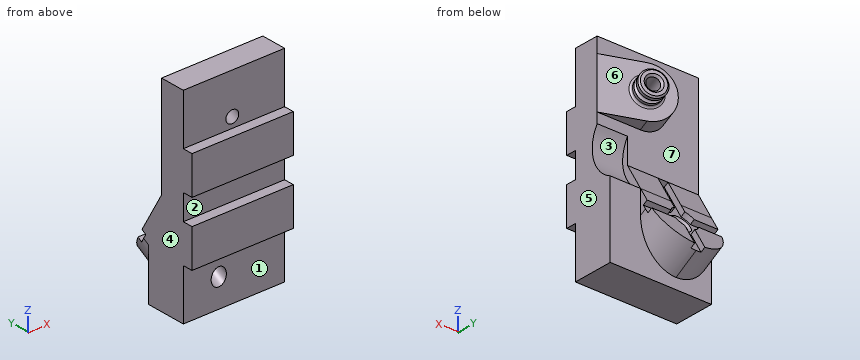
```python
from build123d import *

# Parameters (mm, degrees)
BOSS_EXTRUDE1_DEPTH     = 100
CUT_EXTRUDE1_DEPTH      = 30
BOSS_EXTRUDE2_START     = -15
BOSS_EXTRUDE2_DEPTH     = 50
CUT_EXTRUDE2_REACH      = 226.87
SKETCH5_R               = 12.5
BOSS_EXTRUDE4_DEPTH     = 15
SKETCH7_R               = 6
CUT_EXTRUDE4_DEPTH      = 228.547988513
FILLET1_R               = 2
CHAMFER1_SIZE           = 2
CHAMFER2_SIZE           = 1.5
BOSS_EXTRUDE5_DEPTH     = 70
CUT_EXTRUDE5_REACH      = 232.227
CUT_EXTRUDE6_DEPTH      = 5
CUT_EXTRUDE7_DEPTH      = 230.919504684
CUT_EXTRUDE7_DEPTH_BACK = 230.919504684
SKETCH17_R              = 7.5
CHAMFER3_SIZE           = 2


with BuildPart() as part:
    # Sketch1 → Boss-Extrude1 (new body)
    with BuildSketch(Plane(origin=(0, 0, 0), x_dir=(0, 0, -1), z_dir=(1, 0, 0))):
        Polygon((0, 0), (50, 0), (50, -10), (87.5, -10), (87.5, 0), (112.5, 0), (112.5, -10), (150, -10), (150, 0), (200, 0), (200, 40), (125.980762114, 40), (100, 25), (0, 25), align=None)
    extrude(amount=BOSS_EXTRUDE1_DEPTH)

    # Sketch2 → Cut-Extrude1 (cut)
    with BuildSketch(Plane(origin=(100, 0, 0), x_dir=(0, 0, -1), z_dir=(1, 0, 0))):
        with BuildLine():
            Line((100, 25), (75, 25))
            ThreePointArc((75, 25), (103.939266476, 20.77821286), (125.980762114, 40))
            Line((125.980762114, 40), (100, 25))
        make_face()
    extrude(amount=-CUT_EXTRUDE1_DEPTH, mode=Mode.SUBTRACT)

    # Sketch3 → Boss-Extrude2 (add)
    with BuildSketch(Plane.XY.offset(BOSS_EXTRUDE2_START)):
        Polygon((100, 25), (30.828444789, 25), (38.919979649, 47.231309316), align=None)
    extrude(amount=-BOSS_EXTRUDE2_DEPTH)

    # Cut-Extrude2: up to this plane
    cut_extrude2_end = Plane(origin=(100, 25, 0), z_dir=(0, -1, 0))
    # Sketch4 → Cut-Extrude2 (cut, up to the surface)
    with BuildSketch(Plane(origin=(19.732622965, 54.214936023, 0), x_dir=(0.9396926207859106, -0.3420201433256628, 0), z_dir=(0.34202014332566283, 0.9396926207859106, 0)), mode=Mode.PRIVATE) as cut_extrude2_sk1:
        with BuildLine():
            ThreePointArc((20.418758495, 40), (27.741088966, 57.67766953), (45.418758495, 65))
            Line((45.418758495, 65), (20.418758495, 65))
            Line((20.418758495, 65), (20.418758495, 40))
        make_face()
    cut_extrude2_tool1 = split(extrude(cut_extrude2_sk1.sketch, amount=-CUT_EXTRUDE2_REACH, mode=Mode.PRIVATE), bisect_by=cut_extrude2_end, keep=Keep.BOTH, mode=Mode.PRIVATE)
    add(cut_extrude2_tool1.solids().sort_by_distance((44.16741, 45.321401, -59.415802))[0], mode=Mode.SUBTRACT)
    # Sketch4 → Cut-Extrude2 (cut, up to the surface)
    with BuildSketch(Plane(origin=(19.732622965, 54.214936023, 0), x_dir=(0.9396926207859106, -0.3420201433256628, 0), z_dir=(0.34202014332566283, 0.9396926207859106, 0)), mode=Mode.PRIVATE) as cut_extrude2_sk2:
        with BuildLine():
            ThreePointArc((45.418758495, 15), (27.741088966, 22.32233047), (20.418758495, 40))
            Line((20.418758495, 40), (20.418758495, 15))
            Line((20.418758495, 15), (45.418758495, 15))
        make_face()
    cut_extrude2_tool2 = split(extrude(cut_extrude2_sk2.sketch, amount=-CUT_EXTRUDE2_REACH, mode=Mode.PRIVATE), bisect_by=cut_extrude2_end, keep=Keep.BOTH, mode=Mode.PRIVATE)
    add(cut_extrude2_tool2.solids().sort_by_distance((44.16741, 45.321401, -20.584198))[0], mode=Mode.SUBTRACT)

    # Sketch5 → Boss-Extrude4 (add)
    with BuildSketch(Plane(origin=(19.732622965, 54.214936023, 0), x_dir=(0.9396926207859106, -0.3420201433256628, 0), z_dir=(0.34202014332566283, 0.9396926207859106, 0))):
        with Locations(Location((45.418758495, 40, 0), (0, 0, 180))):
            Circle(SKETCH5_R)
    extrude(amount=BOSS_EXTRUDE4_DEPTH)

    # Sketch7 → Cut-Extrude4 (cut, through all)
    with BuildSketch(Plane(origin=(24.862925115, 68.310325335, 0), x_dir=(0.9396926207859105, -0.3420201433256629, 0), z_dir=(0.34202014332566294, 0.9396926207859106, 0))):
        with Locations(Location((45.418758495, 40, 0), (0, 0, 180))):
            Circle(SKETCH7_R)
    extrude(amount=-CUT_EXTRUDE4_DEPTH, mode=Mode.SUBTRACT)

    # Fillet1
    fillet1_edges = [part.edges().sort_by_distance(p)[0] for p in [
        (74.158452928, 34.405553941, -40),
    ]]
    fillet(fillet1_edges, radius=FILLET1_R)

    # Chamfer1
    chamfer1_edges = [part.edges().sort_by_distance(p)[0] for p in [
        (73.180753043, 50.724074185, -40),
    ]]
    chamfer(chamfer1_edges, length=CHAMFER1_SIZE)

    # Sketch11 → Cut-Revolve1 (revolve, cut)
    with BuildSketch(Plane(origin=(42.679672203, -15.53413029, 0), x_dir=(0.34202014332566294, 0.9396926207859105, 0), z_dir=(0.9396926207859105, -0.342020143325663, 0)), mode=Mode.PRIVATE) as cut_revolve1_sk:
        with BuildLine():
            Line((67.694329852, -27.5), (62.694329852, -27.5))
            ThreePointArc((62.694329852, -27.5), (65.194329852, -30), (67.694329852, -27.5))
        make_face()
    revolve(cut_revolve1_sk.sketch.rotate(Axis((43.396560119, -13.564496931, -40), (0.34202014332566283, 0.9396926207859105, 0)), 90), axis=Axis((43.396560119, -13.564496931, -40), (0.34202014332566283, 0.9396926207859105, 0)), mode=Mode.SUBTRACT)

    # Chamfer2
    chamfer2_edges = [part.edges().sort_by_distance(p)[0] for p in [
        (79.288755078, 48.500943253, -40),
    ]]
    chamfer(chamfer2_edges, length=CHAMFER2_SIZE)

    # Sketch13 → Boss-Extrude5 (add)
    with BuildSketch(Plane.ZY):
        Polygon((-125.980762114, 40), (-173.612159322, 67.5), (-189.489291724, 40), align=None)
    extrude(amount=-BOSS_EXTRUDE5_DEPTH)

    # Cut-Extrude5: up to this plane
    cut_extrude5_end = Plane(origin=(100, 40, -200), z_dir=(0, -1, 0))
    # Sketch14 → Cut-Extrude5 (cut, up to the surface)
    with BuildSketch(Plane(origin=(0, -24.551270189, -14.174682453), x_dir=(1, 0, 0), z_dir=(0, 0.8660254037844378, 0.5000000000000016)), mode=Mode.PRIVATE) as cut_extrude5_sk1:
        with BuildLine():
            Line((70, 184.102540378), (35, 184.102540378))
            ThreePointArc((35, 184.102540378), (59.748737342, 173.85127772), (70, 149.102540378))
            Line((70, 149.102540378), (70, 184.102540378))
        make_face()
    cut_extrude5_tool1 = split(extrude(cut_extrude5_sk1.sketch, amount=-CUT_EXTRUDE5_REACH, mode=Mode.PRIVATE), bisect_by=cut_extrude5_end, keep=Keep.BOTH, mode=Mode.PRIVATE)
    add(cut_extrude5_tool1.solids().sort_by_distance((62.182122, 63.591061, -166.841678))[0], mode=Mode.SUBTRACT)
    # Sketch14 → Cut-Extrude5 (cut, up to the surface)
    with BuildSketch(Plane(origin=(0, -24.551270189, -14.174682453), x_dir=(1, 0, 0), z_dir=(0, 0.8660254037844378, 0.5000000000000016)), mode=Mode.PRIVATE) as cut_extrude5_sk2:
        with BuildLine():
            Line((0, 184.102540378), (0, 149.102540378))
            ThreePointArc((0, 149.102540378), (10.251262658, 173.85127772), (35, 184.102540378))
            Line((35, 184.102540378), (0, 184.102540378))
        make_face()
    cut_extrude5_tool2 = split(extrude(cut_extrude5_sk2.sketch, amount=-CUT_EXTRUDE5_REACH, mode=Mode.PRIVATE), bisect_by=cut_extrude5_end, keep=Keep.BOTH, mode=Mode.PRIVATE)
    add(cut_extrude5_tool2.solids().sort_by_distance((7.817878, 63.591061, -166.841678))[0], mode=Mode.SUBTRACT)

    # Sketch15 → Cut-Extrude6 (cut)
    with BuildSketch(Plane(origin=(0, -24.551270189, -14.174682453), x_dir=(1, 0, 0), z_dir=(0, 0.8660254037844378, 0.5000000000000016))):
        with BuildLine():
            ThreePointArc((40, 183.74355653), (35, 184.102540378), (30, 183.74355653))
            Line((30, 183.74355653), (30, 160.558979616))
            ThreePointArc((30, 160.558979616), (26.161165235, 157.941375143), (23.543560763, 154.102540378))
            Line((23.543560763, 154.102540378), (0.358983849, 154.102540378))
            ThreePointArc((0.358983849, 154.102540378), (0.08986132, 151.608975566), (0, 149.102540378))
            Line((0, 149.102540378), (0, 144.102540378))
            Line((0, 144.102540378), (23.543560763, 144.102540378))
            ThreePointArc((23.543560763, 144.102540378), (26.161165235, 140.263705614), (30, 137.646101141))
            Line((30, 137.646101141), (30, 99.102540378))
            Line((30, 99.102540378), (40, 99.102540378))
            Line((40, 99.102540378), (40, 137.646101141))
            ThreePointArc((40, 137.646101141), (43.838834765, 140.263705614), (46.456439237, 144.102540378))
            Line((46.456439237, 144.102540378), (70, 144.102540378))
            Line((70, 144.102540378), (70, 149.102540378))
            ThreePointArc((70, 149.102540378), (69.91013868, 151.608975566), (69.641016151, 154.102540378))
            Line((69.641016151, 154.102540378), (46.456439237, 154.102540378))
            ThreePointArc((46.456439237, 154.102540378), (43.838834765, 157.941375143), (40, 160.558979616))
            Line((40, 160.558979616), (40, 183.74355653))
        make_face()
    extrude(amount=-CUT_EXTRUDE6_DEPTH, mode=Mode.SUBTRACT)

    # Sketch17 → Cut-Extrude7 (cut, two sides: drawn at the far end of the back side and taken through both)
    with BuildSketch(Plane(origin=(0, -28.881397208, -16.674682453), x_dir=(1, 0, 0), z_dir=(0, 0.8660254037844378, 0.5000000000000016)).offset(-CUT_EXTRUDE7_DEPTH_BACK)):
        with Locations(Location((35, 149.102540378, 0), (0, 0, 270))):
            Circle(SKETCH17_R)
    extrude(amount=CUT_EXTRUDE7_DEPTH + CUT_EXTRUDE7_DEPTH_BACK, mode=Mode.SUBTRACT)

    # Chamfer3
    chamfer3_edges = [part.edges().sort_by_distance(p)[0] for p in [
        (35, 49.419872981, -152.296460718),
    ]]
    chamfer(chamfer3_edges, length=CHAMFER3_SIZE)


solid = part.part
```
Geometry check sheet. Reference: the model listing, model coordinates, mm. Face numbers are marked on the shaded views. A direction names the side the tool comes from. Round coordinates to 2 decimals unless told otherwise and drop trailing zeros. Loops run counter-clockwise (first coordinate to the right, second up) from the corner with the lowest first, then second, coordinate; pieces in that order, holes last. Notation, with made-up numbers: (64.25, 65) - (68.25, 65) arc R22 ccw to (68.25, 86) - close; hole circle Ø1 at (71, -2.5). An arc over 180 degrees is marked (long way). Use a Markdown table: item, result.
Q1. Access from +Z, -Z, +X, -X, +Y, -Y to the whole of each face (thin tool, end or side, straight path). Record for the marked faces 1, 2 and 3.
Solutions:
| item | result |
|---|---|
| face 1 | -Z, +X, -X, -Y |
| face 2 | +X, -X, -Y |
| face 3 | +X, +Y |
Q2. Material ranges on line 1 (Z direction, x = 85.5, y = -3); line 2 (X direction, y = 28, z = -109.5); line 3 (Z direction, x = 52, y = 25.5), recorded low to high.
Solutions:
| item | result |
|---|---|
| line 1 | z = -150 to -112.5, -87.5 to -50 |
| line 2 | x = 0 to 30, 40 to 70 |
| line 3 | z = -200 to -100.87, -64.44 to -42.86, -37.14 to -15.56 |
Q3. Cross-section at D-D on z = -93. Record the cut outline in (x, y), plus the area to 3 significant figures.
Solutions:
| item | result |
|---|---|
| outline | (0, 0) - (100, 0) - (100, 19.37) - (70, 19.37) - (70, 25) - (0, 25) - close |
| area | 2,330 mm2 |
Q4. Go/stop test with flat-tipped pins: P1, Ø25, axis at x = 37, z = -167.5, coming from the -Y side; P2, Ø4, axis at x = 56, y = 51, coming from the +Z side; P3, Ø4, axis at x = 33.5, z = -138, coming from the +Y side. Record where each tip stops, or that it passes through.
Solutions:
| item | result |
|---|---|
| P1 | stops at y = 0 |
| P2 | stops at z = -30.69 |
| P3 | stops at y = 41.25 |
Q5. Cross-section at C-C on y = 28. State how many separate pieces and enclosed holes the cut face has, plus the area to 3 significant figures.
Solutions:
| item | result |
|---|---|
| separate pieces | 2 |
| enclosed holes | 2 |
| area | 11,400 mm2 |
Q6. Cross-section at A-A on y = -3.5. Record the cut outline in (x, z).
Solutions:
| item | result |
|---|---|
| outline | (0, -150) - (100, -150) - (100, -112.5) - (0, -112.5) - close; (0, -87.5) - (100, -87.5) - (100, -50) - (0, -50) - close |
Q7. Draft check along X on the marked faces 4, 5, 6 and 7. Enter one of: released by +X, released by -X, zero draft, split by the parting line, or undercut.
Solutions:
| item | result |
|---|---|
| face 4 | released by -X |
| face 5 | released by +X |
| face 6 | undercut |
| face 7 | zero draft |
Q8. Cross-section at B-B on x = 12. Record the cut outline in (y, z).
Solutions:
| item | result |
|---|---|
| outline | (-10, -150) - (0, -150) - (0, -200) - (40, -200) - (40, -179.54) - (63.19, -166.15) - (52.5, -147.63) - (48.17, -150.13) - (43.17, -141.47) - (47.5, -138.97) - (25, -100) - (25, 0) - (0, 0) - (0, -50) - (-10, -50) - (-10, -87.5) - (0, -87.5) - (0, -112.5) - (-10, -112.5) - close |
